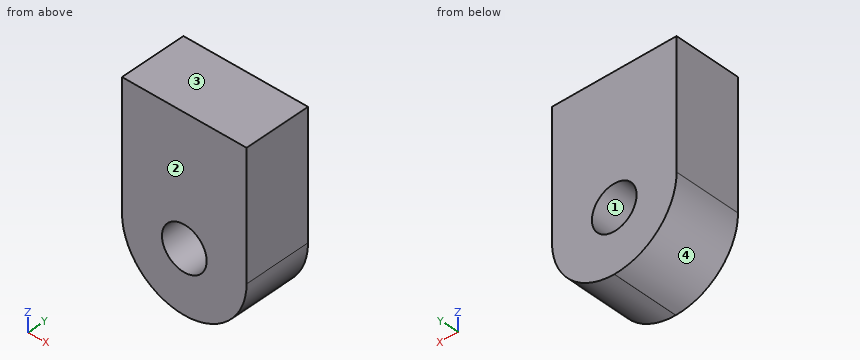
```python
from build123d import *

# Parameters (mm, degrees)
SKETCH1_R           = 5.565
BOSS_EXTRUDE1_DEPTH = 16.59


with BuildPart() as part:
    # Sketch1 → Boss-Extrude1 (new body)
    with BuildSketch(Plane(origin=(0, 0, 0), x_dir=(1, 0, 0), z_dir=(0, 1, 0))):
        with BuildLine():
            Line((0, 0), (31.05, 0))
            Line((31.05, 0), (31.05, 31.62))
            ThreePointArc((31.05, 31.62), (26.504297244, 42.594297244), (15.53, 47.14))
            Line((15.53, 47.14), (15.52, 47.14))
            ThreePointArc((15.52, 47.14), (4.545702756, 42.594297244), (0, 31.62))
            Line((0, 31.62), (0, 0))
        make_face()
        with Locations((15.53, 31.62)):
            Circle(SKETCH1_R, mode=Mode.SUBTRACT)
    extrude(amount=BOSS_EXTRUDE1_DEPTH)


solid = part.part
```
Part model, mm, in its own coordinate system. Face numbers are marked on the shaded views. Coordinates: 2 decimals unless noted, no trailing zeros. Loops run counter-clockwise (first coordinate to the right, second up) from the corner with the lowest first, then second, coordinate; pieces in that order, holes last. Notation, with made-up numbers: (46.25, 86) - (80.25, 86) arc R18 cw to (80.25, 118) - close; hole circle Ø5 at (87.25, 79). An arc over 180 degrees is marked (long way). Write item = value, one per line. Start each with the question number.
Item 1: Cut at D-D, the plane x = 3.5. Give the cut face in (y, z).
Item 2: Cut at B-B, the plane z = -36. Give the cut face in (x, y), and give its area (3 significant figures).
Item 3: Cut at A-A, the plane y = 14.75. Give the cut face in (x, z) (3 decimals).
Item 4: Wall check: L1, parallel to X at y = 9.5, z = -31.62 (3 decimals); L2, parallel to X at y = 1, z = -27; L3, parallel to Z at x = 11.5, y = 4.25. Give the ranges that are in metal, low to high. Write a range as from..to.
Item 5: Mould opens along Z. For the marked faces 1, 2, 3 and 4 say: released by +Z, released by -Z, zero draft, split by the parting line, or undercut.
Item 6: Cut at C-C, the plane x = 14.5. Give the cut face in (y, z), and give its area (3 significant figures).
The answers:
q1.outline = (0, -41.44) - (16.59, -41.44) - (16.59, 0) - (0, 0) - close
q2.outline = (0.63, 0) - (12.1, 0) - (12.1, 16.59) - (0.63, 16.59) - close; (18.96, 0) - (30.42, 0) - (30.42, 16.59) - (18.96, 16.59) - close
q2.area = 380 mm2
q3.outline = (0, -31.62) arc R15.52 ccw to (15.52, -47.14) - (15.53, -47.14) arc R15.52 ccw to (31.05, -31.62) - (31.05, 0) - (0, 0) - close; hole circle Ø11.13 at (15.53, -31.62)
q4.L1 = 0..9.965, 21.095..31.05
q4.L2 = 0..12.43, 18.63..31.05
q4.L3 = -46.61..-35.46, -27.78..0
q5.face_1 = undercut
q5.face_2 = zero draft
q5.face_3 = released by +Z
q5.face_4 = released by -Z
q6.outline = (0, -47.11) - (16.59, -47.11) - (16.59, -37.09) - (0, -37.09) - close; (0, -26.15) - (16.59, -26.15) - (16.59, 0) - (0, 0) - close
q6.area = 600 mm2
